```python
from build123d import *

# Parameters (mm, degrees)
SKETCH_1_R          = 5.0225
SKETCH_1_R_2        = 2.05
EXTRUDE_1_DEPTH     = 2
FILLET_1_R          = 2
FILLET_2_R          = 1.3
SKETCH_3_R          = 5
CUT_EXTRUDE_1_DEPTH = 2


with BuildPart() as part:
    # 草图1 → 凸台-拉伸1 (new body)
    with BuildSketch(Plane.XY):
        with BuildLine():
            Line((298.545628784, -83.894391363), (298.545628784, -92.841778663))
            Line((298.545628784, -92.841778663), (302.545628784, -92.841778663))
            Line((302.545628784, -92.841778663), (302.545628784, -91.391778663))
            Line((302.545628784, -91.391778663), (305.745628784, -91.391778663))
            Line((305.745628784, -91.391778663), (305.745628784, -92.841778663))
            Line((305.745628784, -92.841778663), (308.945628784, -92.841778663))
            Line((308.945628784, -92.841778663), (308.945628784, -96.941778663))
            Line((308.945628784, -96.941778663), (305.745628784, -96.941778663))
            Line((305.745628784, -96.941778663), (305.745628784, -98.391778663))
            Line((305.745628784, -98.391778663), (302.545628784, -98.391778663))
            Line((302.545628784, -98.391778663), (302.545628784, -96.941778663))
            Line((302.545628784, -96.941778663), (298.545628784, -96.941778663))
            Line((298.545628784, -96.941778663), (298.545628784, -105.894391358))
            Line((298.545628784, -105.894391358), (293.545628784, -105.894391358))
            Line((293.545628784, -105.894391358), (293.545628784, -113.894391358))
            Line((293.545628784, -113.894391358), (298.545628784, -113.894391358))
            Line((298.545628784, -113.894391358), (298.545628784, -122.847004054))
            Line((298.545628784, -122.847004054), (302.545628784, -122.847004054))
            Line((302.545628784, -122.847004054), (302.545628784, -121.397004054))
            Line((302.545628784, -121.397004054), (305.745628784, -121.397004054))
            Line((305.745628784, -121.397004054), (305.745628784, -122.847004054))
            Line((305.745628784, -122.847004054), (308.945628784, -122.847004054))
            Line((308.945628784, -122.847004054), (308.945628784, -126.947004054))
            Line((308.945628784, -126.947004054), (305.745628784, -126.947004054))
            Line((305.745628784, -126.947004054), (305.745628784, -128.397004054))
            Line((305.745628784, -128.397004054), (302.545628784, -128.397004054))
            Line((302.545628784, -128.397004054), (302.545628784, -126.947004054))
            Line((302.545628784, -126.947004054), (298.545628784, -126.947004054))
            Line((298.545628784, -126.947004054), (298.545628784, -140.447004054))
            Line((298.545628784, -140.447004054), (324.188862368, -140.447004054))
            Line((324.188862368, -140.447004054), (376.358604426, -71.946984141))
            Line((376.358604426, -71.946984141), (376.358604426, 4.396201153))
            ThreePointArc((376.358604426, 4.396201153), (348.536987634, 32.217817945), (320.715370843, 4.396201153))
            Line((320.715370843, 4.396201153), (307.936987634, -35.346984141))
            Line((307.936987634, -35.346984141), (298.545628784, -35.346984141))
            Line((298.545628784, -35.346984141), (298.545628784, -45.889165972))
            Line((298.545628784, -45.889165972), (293.545628784, -45.889165972))
            Line((293.545628784, -45.889165972), (293.545628784, -53.889165972))
            Line((293.545628784, -53.889165972), (298.545628784, -53.889165972))
            Line((298.545628784, -53.889165972), (298.545628784, -62.841778668))
            Line((298.545628784, -62.841778668), (302.545628784, -62.841778668))
            Line((302.545628784, -62.841778668), (302.545628784, -61.391778668))
            Line((302.545628784, -61.391778668), (305.745628784, -61.391778668))
            Line((305.745628784, -61.391778668), (305.745628784, -62.841778668))
            Line((305.745628784, -62.841778668), (308.945628784, -62.841778668))
            Line((308.945628784, -62.841778668), (308.945628784, -66.941778668))
            Line((308.945628784, -66.941778668), (305.745628784, -66.941778668))
            Line((305.745628784, -66.941778668), (305.745628784, -68.391778668))
            Line((305.745628784, -68.391778668), (302.545628784, -68.391778668))
            Line((302.545628784, -68.391778668), (302.545628784, -66.941778668))
            Line((302.545628784, -66.941778668), (298.545628784, -66.941778668))
            Line((298.545628784, -66.941778668), (298.545628784, -75.894391363))
            Line((298.545628784, -75.894391363), (293.545628784, -75.894391363))
            Line((293.545628784, -75.894391363), (293.545628784, -83.894391363))
            Line((293.545628784, -83.894391363), (298.545628784, -83.894391363))
        make_face()
        with Locations((348.536987634, 4.396201153)):
            Circle(SKETCH_1_R, mode=Mode.SUBTRACT)
        with Locations((320.545628784, -134.447004054)):
            Circle(SKETCH_1_R_2, mode=Mode.SUBTRACT)
        with Locations((370.358604426, -65.946984141)):
            Circle(SKETCH_1_R_2, mode=Mode.SUBTRACT)
        with Locations((313.936987634, -41.346984141)):
            Circle(SKETCH_1_R_2, mode=Mode.SUBTRACT)
        Polygon((354.947285032, -70.136765586), (328.579617375, -106.396108383), (325.08144343, -57.115165973), align=None, mode=Mode.SUBTRACT)
        Polygon((329.571126451, -37.254352656), (354.337315751, -48.052488042), (344.758747766, -17.175445836), align=None, mode=Mode.SUBTRACT)
    extrude(amount=EXTRUDE_1_DEPTH)

    # 圆角1
    fillet_1_edges = [part.edges().sort_by_distance(p)[0] for p in [
        (354.947285032, -70.136765586, 1),
        (325.08144343, -57.115165973, 1),
        (328.579617375, -106.396108383, 1),
        (344.758747766, -17.175445836, 1),
        (329.571126451, -37.254352656, 1),
        (354.337315751, -48.052488042, 1),
    ]]
    fillet(fillet_1_edges, radius=FILLET_1_R)

    # 圆角2
    fillet_2_edges = [part.edges().sort_by_distance(p)[0] for p in [
        (293.545628784, -113.894391358, 1),
        (293.545628784, -105.894391358, 1),
        (293.545628784, -83.894391363, 1),
        (293.545628784, -75.894391363, 1),
        (293.545628784, -53.889165972, 1),
        (293.545628784, -45.889165972, 1),
    ]]
    fillet(fillet_2_edges, radius=FILLET_2_R)

    # 草图3 → 切除-拉伸1 (cut)
    with BuildSketch(Plane(origin=(0, 0, 0), x_dir=(-1, 0, 0), z_dir=(0, 0, -1))):
        with Locations((-309.899887982, -29.241993317)):
            Circle(SKETCH_3_R)
    extrude(amount=-CUT_EXTRUDE_1_DEPTH, mode=Mode.SUBTRACT)


solid = part.part
```
Source: CAD feature listing. Evaluate the final solid. Frame: model axes, mm. A direction names the side the tool comes from. Round coordinates to 2 decimals unless told otherwise and drop trailing zeros. Loops run counter-clockwise (first coordinate to the right, second up) from the corner with the lowest first, then second, coordinate; pieces in that order, holes last. Notation, with made-up numbers: M -23,8 L -10,8 A26 cw -10,30 Z; hole C 50.5,26 d1. An arc over 180 degrees is marked long. Use a Markdown table: item, result. Add a question column.
1. Cut plane A-A, the plane x = 339. Output: boundary loops of the cut face in (y, z).
2. Contact query for flat-ended pins moving along their axis: pin 1 (0.6 mm diameter, centred on x = 303.5, z = 1.5, fed in from +Y); pin 2 (0.6 mm diameter, centred on y = -88, z = 1, fed in from -X); pin 3 (0.6 mm diameter, centred on x = 296.5, z = 1.5, fed in from +Y). Output: stop coordinate, or through.
3. Cut plane C-C, the plane x = 347.5. Output: boundary loops of the cut face in (y, z), and give its area (3 significant figures).
4. Ray query, line 1 along Y through (x, z) = (298.5, 1.6); line 2 along Y through (x, z) = (306.5, 0.6); line 3 along Y through (x, z) = (341, 1.3). Return the intervals inside material, ascending. Write a range as [from, to].
5. Set-up query: faces 5 (the flat face through (334, -53, 0)), 6 (the flat face through (349.53, -32.55, 0.99)). Return all of +Z, -Z, +X, -X, +Y, -Y with unobstructed straight access to the full face (end or side cutting, diameter ignored); none if empty.
6. Cut plane D-D, the plane z = 0.95. State how many separate pieces and enclosed holes the cut face has, and give its area (3 significant figures).
7. Cut plane B-B, the plane y = -31.5. Output: boundary loops of the cut face in (x, z), and give its area (3 significant figures).
8. Pull-direction query (X, two-part tool) for faces 1 (the flat face through (316.14, -9.84, 0.99)), 2 (the flat face through (340.987, -42.232, 0.986)), 3 (the cylindrical face through (349.15, 32.21, 0.99)), 4 (the cylindrical face through (314.69, -30.67, 0.99)); classes: +X half, -X half, draft (parallel to the pull), parting line (faces both ways), or undercut.
Solution:
| question | item | result |
|---|---|---|
| 1 | outline | M -121,0 L -92.07,0 L -92.07,2 L -121,2 Z; M -63.18,0 L -41.37,0 L -41.37,2 L -63.18,2 Z; M -24.79,0 L 30.53,0 L 30.53,2 L -24.79,2 Z |
| 2 | pin 1 | stops at y = -35.35 |
| 2 | pin 2 | stops at x = 298.55 |
| 2 | pin 3 | stops at y = -45.89 |
| 3 | outline | M -109.84,0 L -80.38,0 L -80.38,2 L -109.84,2 Z; M -66.89,0 L -45.07,0 L -45.07,2 L -66.89,2 Z; M -26.01,0 L -0.52,0 L -0.52,2 L -26.01,2 Z; M 9.31,0 L 32.2,0 L 32.2,2 L 9.31,2 Z |
| 3 | area | 199 mm2 |
| 4 | line 1 | y = [-113.89, -105.89], [-83.89, -75.89], [-53.89, -45.89] |
| 4 | line 2 | y = [-140.45, -126.95], [-122.85, -96.94], [-92.84, -66.94], [-62.84, -35.35] |
| 4 | line 3 | y = [-118.37, -89.32], [-64.06, -42.24], [-22.14, 31.18] |
| 5 | face 5 | -Z, +X, -X, +Y, -Y |
| 5 | face 6 | +Z, -Z |
| 6 | separate pieces | 1 |
| 6 | enclosed holes | 6 |
| 6 | area | 8,850 mm2 |
| 7 | outline | M 314.36,0 L 333.92,0 L 333.92,2 L 314.36,2 Z; M 349.2,0 L 376.36,0 L 376.36,2 L 349.2,2 Z |
| 7 | area | 93.4 mm2 |
| 8 | face 1 | -X half |
| 8 | face 2 | undercut |
| 8 | face 3 | parting line |
| 8 | face 4 | undercut |
